Geometry: final body of the model. Coordinates: model frame, mm. Face numbers are marked on the shaded views. A direction names the side the tool comes from. Round coordinates to 2 decimals unless told otherwise and drop trailing zeros. Order: outer loops, then holes, each group sorted by start corner. A loop starts at its lowest first (then second) coordinate and runs counter-clockwise, first axis right, second up. Notation, with made-up numbers: (63.25, 49) -> (117.25, 49) arc R30 cw to (117.25, 75) -> close; hole circle Ø10 at (61.25, 79). An arc over 180 degrees is marked (long way). Put each result on its own line as item: value.
```python
from build123d import *

# Parameters (mm, degrees)
F0_W     = 100
F0_H     = 100
F0_W_2   = 40
F0_H_2   = 40
F1_DEPTH = 20
F3_DEPTH = 15


with BuildPart() as f1:
    # F0 (on Front) → F1 (new body)
    with BuildSketch(Plane.XZ):
        Rectangle(F0_W, F0_H)
        Rectangle(F0_W_2, F0_H_2, mode=Mode.SUBTRACT)
    extrude(amount=F1_DEPTH)

    # F2 (on Right) → F3 (join, symmetric)
    with BuildSketch(Plane.YZ):
        Polygon((80, -28.63813), (0, 51.36187), (0, -28.63813), align=None)
    extrude(amount=F3_DEPTH, both=True)


solid = f1.part
```
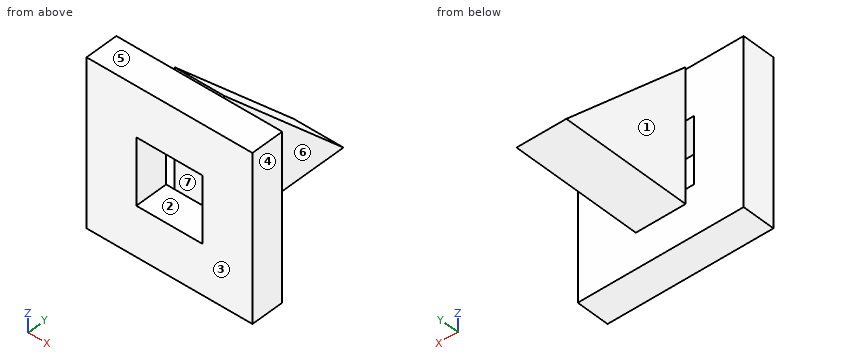
1. Cut plane A-A on z = -3.5. Return loops of the section in (x, y).
Ans:
outline: (-50, -20) -> (-20, -20) -> (-20, 0) -> (-50, 0) -> close; (-15, 0) -> (15, 0) -> (15, 54.86) -> (-15, 54.86) -> close; (20, -20) -> (50, -20) -> (50, 0) -> (20, 0) -> close
2. Set-up query: the marked faces 5, 6 and 7. Return all of +Z, -Z, +X, -X, +Y, -Y with unobstructed straight access to the full face (end or side cutting, diameter ignored); none if empty.
Ans:
face 5: +Z, +X, -X, -Y
face 6: +Z, -Z, +X, +Y
face 7: -Y
3. Draft query along X for the marked faces 1, 2, 3 and 4. Return one class per face: +X half, -X half, draft (parallel to the pull), parting line (faces both ways), or undercut.
Ans:
face 1: -X half
face 2: undercut
face 3: draft
face 4: +X half
4. Cut plane B-B on x = 16.5. Return loops of the section in (y, z).
Ans:
outline: (-20, -50) -> (0, -50) -> (0, -20) -> (-20, -20) -> close; (-20, 20) -> (0, 20) -> (0, 50) -> (-20, 50) -> close
5. Cut plane D-D on y = 48.5. Return loops of the section in (x, z), and give its area (3 significant figures).
Ans:
outline: (-15, -28.64) -> (15, -28.64) -> (15, 2.86) -> (-15, 2.86) -> close
area: 945 mm²
6. Cut plane C-C on x = -13. Return loops of the section in (y, z), and give its area (3 significant figures).
Ans:
outline: (-20, -50) -> (0, -50) -> (0, -28.64) -> (80, -28.64) -> (0, 51.36) -> (0, 50) -> (-20, 50) -> (-20, 20) -> (0, 20) -> (0, -20) -> (-20, -20) -> close
area: 4,400 mm²
7. Material intervals for probe 1 along X at (y, z) = (-10, -12.5); probe 2 along X at (y, z) = (70, -21.5); probe 3 along Y at (x, z) = (-30, 4), sorted ascending.
Ans:
probe 1: -50 to -20, 20 to 50
probe 2: -15 to 15
probe 3: -20 to 0
8. Contact query for flat-ended pins moving along their axis: P1, Ø10, axis at x = 1, y = -10.5, coming from the +Z side; P2, Ø15, axis at x = -6.5, z = 1.5, coming from the -Y side; P3, Ø1.5, axis at x = -11.5, y = 40, coming from the +Z side; P4, Ø5, axis at y = 1.5, z = 16, coming from the -X side. Output: stop coordinate, or through.
Ans:
P1: z = 50
P2: y = 0
P3: z = 12.11
P4: x = -50
